Autodesk Inventor part; units mm, degrees
ref_plane "Work Plane1" through (0, 80, 0) normal (-0.7071, 0, 0.7071) x (0, -1, 0)
ref_plane "YZ Plane" through (0, 0, 0) normal (1, 0, 0) x (0, 1, 0)
ref_plane "XZ Plane" through (0, 0, 0) normal (0, 1, 0) x (-1, 0, 0)
sketch "Sketch1" plane through (0, 0, 0) normal (0, 0, 1) x (1, 0, 0)
  line L0 (0, 0) -> (200, 0)
  line L1 (200, 0) -> (200, 80)
  line L2 (200, 80) -> (0, 80)
  line L3 (0, 80) -> (0, 0)
  dimension "d0" = 200
  dimension "d1" = 80
extrude "Extrusion1" add sketch "Sketch1" along normal blind 200
sketch "Sketch2" plane through (0, 80, 0) normal (0, 1, 0) x (1, 0, 0)
  line L0 (0, 0) -> (200, 0)
  line L1 (0, 0) -> (0, -200)
  line L2 (10, -20.6066) -> (10, -190)
  line L3 (20.6066, -10) -> (190, -10)
  line L4 (10, -20.6066) -> (10, -25)
  line L5 (20.6066, -10) -> (25, -10)
  line L6 (105.3033, -94.6967) -> (20.6066, -10)
  line L7 (94.6967, -105.3033) -> (10, -20.6066)
  line L8 (190, -10) -> (105.3033, -94.6967)
  line L9 (94.6967, -105.3033) -> (10, -190)
  line L10 (105.3033, -73.4835) -> (153.7868, -25)
  line L11 (94.6967, -105.3033) -> (84.0901, -115.9099)
  line L12 (73.4835, -105.3033) -> (25, -56.8198)
  line L13 (105.3033, -73.4835) -> (56.8198, -25)
  line L14 (153.7868, -25) -> (56.8198, -25)
  line L15 (25, -56.8198) -> (25, -153.7868)
  line L16 (134.3503, -134.3503) -> (91.9239, -176.7767)
  line L17 (63.6396, -148.4924) -> (148.4924, -63.6396)
  line L18 (176.7767, -91.9239) -> (134.3503, -134.3503)
  arc A0 (176.7767, -91.9239) -> (148.4924, -63.6396) centre (162.6346, -77.7817) ccw
  arc A1 (169.7056, -84.8528) -> (155.5635, -70.7107) centre (162.6346, -77.7817) ccw
  line L19 (169.7056, -84.8528) -> (97.1003, -157.4582)
  line L20 (155.5635, -70.7107) -> (82.9581, -143.316)
  line L21 (73.4835, -105.3033) -> (25, -153.7868)
  line L22 (10, -110.6066) -> (25, -110.6066)
  circle A2 centre (17.5, -110.6066) radius 5.5
  circle A3 centre (17.5, -135.6066) radius 5.5
  circle A4 centre (17.5, -85.6066) radius 5.5
  circle A5 centre (17.5, -65.6066) radius 3.5
  circle A6 centre (17.5, -155.6066) radius 3.5
  arc A7 (63.6396, -148.4924) -> (91.9239, -176.7767) centre (77.7817, -162.6346) ccw
  arc A8 (97.1003, -157.4582) -> (82.9581, -143.316) centre (77.7817, -162.6346) ccw
  dimension "d20" = 40
  dimension "d22" = 11
  dimension "d24" = 11
  dimension "d26" = 11
  dimension "d29" = 7
  dimension "d30" = 7
extrude "Extrusion2" add sketch "Sketch2" along normal blind 10
ref_plane "Work Plane1" through (0, 80, 0) normal (-0.7071, 0, 0.7071) x (0, -1, 0)
sketch "Sketch3" plane through (0, 80, 0) normal (-0.7071, 0, 0.7071) x (0, -1, 0)
  line L0 (80, 282.8427) -> (0, 282.8427)
  line L1 (0, 282.8427) -> (0, 207.8427)
  line L2 (0, 141.4214) -> (0, 282.8427)
  line L3 (0, 282.8427) -> (60, 282.8427)
  line L4 (60, 282.8427) -> (0, 207.8427)
  point P0 (80, 0)
  dimension "d33" = 75
  dimension "d34" = 60
extrude "Extrusion3" cut sketch "Sketch3" along normal mid plane 200
fillet "Fillet1" radius 5 3 edges at (25, 85, 56.8198) (73.4835, 85, 105.3033) (25, 85, 153.7868)
sketch "Sketch5" plane through (0, 90, 0) normal (0, 1, 0) x (1, 0, 0)
  point P0 (0, 0)
sketch "Sketch6" plane through (0, 90, 0) normal (0, 1, 0) x (1, 0, 0)
  arc A0 (63.6396, -148.4924) -> (91.9239, -176.7767) centre (77.7817, -162.6346) ccw
  arc A1 (63.6396, -148.4924) -> (91.9239, -176.7767) centre (77.7817, -162.6346) ccw
  arc A2 (169.7056, -84.8528) -> (155.5635, -70.7107) centre (162.6346, -77.7817) ccw
  arc A3 (176.7767, -91.9239) -> (148.4924, -63.6396) centre (162.6346, -77.7817) ccw
  line L0 (148.4924, -63.6396) -> (63.6396, -148.4924)
  line L1 (63.6396, -148.4924) -> (148.4924, -63.6396)
  line L2 (91.9239, -176.7767) -> (176.7767, -91.9239)
  line L3 (91.9239, -176.7767) -> (176.7767, -91.9239)
  point P0 (0, 0)
extrude "Extrusion5" cut sketch "Sketch6" against normal blind 10
sketch "Sketch7" plane through (0, 90, 0) normal (0, 1, 0) x (1, 0, 0)
  line L0 (105.3033, -94.6967) -> (20.6066, -10)
  line L1 (20.6066, -10) -> (105.3033, -94.6967)
  line L2 (190, -10) -> (105.3033, -94.6967)
  line L3 (105.3033, -94.6967) -> (190, -10)
  line L4 (190, -10) -> (20.6066, -10)
  point P0 (0, 0)
extrude "Extrusion6" cut sketch "Sketch7" against normal blind 10
sketch "Sketch8" plane through (0, 80, 0) normal (0, 1, 0) x (1, 0, 0)
  line L0 (200, 0) -> (0, 0)
  line L1 (0, 0) -> (20.645, 0)
  line L2 (20.645, 0) -> (20.645, -20)
  line L3 (20.645, -20) -> (126.7111, -126.066)
  line L4 (20.645, -20) -> (170.645, -20) construction
  line L5 (126.7111, -126.066) -> (200, -52.7771)
  line L6 (200, 0) -> (200, -93.934)
  line L7 (20.645, 0) -> (200, 0)
  line L8 (200, -52.7771) -> (200, 0)
  dimension "d45" = 20
  dimension "d46" = 150
  dimension "d47" = 45
extrude "Extrusion7" cut sketch "Sketch8" against normal blind 10
fillet "Fillet2" radius 20 2 edges at (126.7111, 75, 126.066) (20.645, 75, 20)
sketch "Sketch9" plane through (0, 70, 0) normal (0, 1, 0) x (1, 0, 0)
  arc A0 (112.5689, -111.9239) -> (140.8532, -111.9239) centre (126.7111, -97.7817) ccw
  arc A1 (117.4902, -106.2213) -> (135.9319, -106.2213) centre (126.7111, -97.7817) ccw
  arc A2 (20.645, -11.7157) -> (26.5029, -25.8579) centre (40.645, -11.7157) ccw
  arc A3 (28.145, -11.7157) -> (31.8071, -20.5555) centre (40.645, -11.7157) ccw
  line L0 (117.4902, -106.2213) -> (31.8071, -20.5555)
  line L1 (135.9319, -106.2213) -> (226.547, -106.2213) construction
  line L2 (200, 0) -> (200, -52.7771)
  line L3 (200, 0) -> (192.5, 0)
  line L4 (20.645, 0) -> (200, 0)
  line L5 (192.5, -7.5) -> (192.5, -49.6532)
  line L6 (200, 0) -> (200, -7.5)
  line L7 (192.5, -7.5) -> (28.145, -7.5)
  line L8 (28.145, -11.7157) -> (28.145, -7.5)
  line L9 (135.9319, -106.2213) -> (192.5, -49.6532)
  line L10 (200, -42.1532) -> (200.0065, -42.1467)
  line L11 (126.7111, -97.7817) -> (126.7111, -85.2817)
  circle A4 centre (126.7111, -97.7817) radius 12.5
  point P0 (0, 0)
  dimension "d51" = 25
  dimension "d52" = 25
  dimension "d54" = 7.5
  dimension "d55" = 7.5
extrude "Extrusion8" cut sketch "Sketch9" against normal blind 10 contours L0 A3 L8 L7 L5 L9 A4
sketch "Sketch10" plane through (0, 70, 0) normal (0, 1, 0) x (1, 0, 0)
  arc A0 (135.9319, -106.2213) -> (117.4902, -106.2213) centre (126.7111, -97.7817) ccw
  circle A1 centre (126.7111, -97.7817) radius 20
  point P0 (0, 0)
extrude "Extrusion9" add sketch "Sketch10" along normal blind 10 and the other way blind 10
sketch "Sketch11" plane through (0, 80, 200) normal (0, 1, 0) x (1, 0, 0)
  arc A0 (146.5879, 104.4347) -> (106.834, 104.4327) centre (126.7111, 102.2183) ccw
  line L0 (126.7111, 102.2183) -> (112.5689, 116.3604)
  line L1 (126.7111, 102.2183) -> (146.7111, 102.2183) construction
  line L2 (112.5689, 116.3604) -> (98.4268, 102.2183)
  line L3 (112.5689, 88.0761) -> (26.5029, 174.1421)
  line L4 (140.8532, 116.3604) -> (154.9953, 102.2183)
  line L5 (200, 147.2229) -> (140.8532, 88.0761)
  arc A1 (112.5689, 88.0761) -> (140.8532, 88.0761) centre (126.7111, 102.2183) ccw
  arc A2 (140.8532, 116.3604) -> (112.5689, 116.3604) centre (126.7111, 102.2183) ccw
  line L6 (112.5689, 88.0761) -> (98.4268, 102.2183)
  line L7 (154.9953, 102.2183) -> (140.8532, 88.0761)
  point P0 (0, 200)
  dimension "d62" = 135
extrude "Extrusion10" add sketch "Sketch11" against normal blind 20
fillet "Fillet3" radius 10 2 edges at (103.7373, 65, 92.4712) (149.6834, 65, 92.4698)
sketch "Sketch12" plane through (0, 70, 0) normal (0, 1, 0) x (1, 0, 0)
  arc A0 (140.8532, -83.6396) -> (112.5689, -83.6396) centre (126.7111, -97.7817) ccw
  line L0 (107.8365, -77.7817) -> (93.1316, -92.4866)
  line L1 (98.4268, -97.7817) -> (26.5029, -25.8579)
  line L2 (146.1565, -78.3363) -> (160.2986, -92.4784)
  line L3 (200, -52.7771) -> (154.9953, -97.7817)
  line L4 (160.2986, -92.4784) -> (127.5069, -125.2702)
  line L5 (127.5069, -125.2702) -> (93.9274, -91.6908)
  arc A1 (146.1565, -78.3363) -> (106.7111, -78.9072) centre (126.7111, -97.7817) ccw
  point P0 (0, 0)
extrude "Extrusion11" add sketch "Sketch12" against normal blind 20 contours A1 L2 L3 L4 L5 L0
fillet "Fillet4" radius 5 2 edges at (98.6681, 65, 86.9501) (154.7622, 65, 86.942)
fillet "Fillet5" radius 5 2 edges at (98.4268, 75, 97.7817) (154.9953, 75, 97.7817)
fillet "Fillet6" radius 5 3 edges at (192.5, 65, 7.5) (192.5, 65, 49.6532) (28.145, 65, 7.5)
sketch "Sketch13" plane through (0, 60, 0) normal (0, 1, 0) x (1, 0, 0)
  line L0 (200, 0) -> (200, -52.7771)
  line L1 (200, 0) -> (200, -35)
  line L2 (200, -35) -> (160, -35)
  circle A0 centre (160, -35) radius 20
  circle A1 centre (160, -35) radius 10
  point P0 (0, 0)
  dimension "d72" = 35
  dimension "d73" = 40
  dimension "d74" = 40
  dimension "d75" = 20
extrude "Extrusion12" add sketch "Sketch13" along normal blind 20
fillet "Fillet7" radius 10 3 edges at (94.6967, 85, 105.3033) (10, 85, 20.6066) (10, 85, 190)
fillet "Fillet8" radius 3 6 edges at (28.0866, 80, 146.3351) (51.7417, 80, 127.045) (71.4124, 80, 105.3033) (51.7417, 80, 83.5616) (28.0866, 80, 64.2715) (25, 80, 105.3033)
sketch "Sketch14" plane through (160, 80, 35) normal (0, 1, 0) x (1, 0, 0)
  circle A0 centre (0, 0) radius 20
  circle A1 centre (-20, 0) radius 5.5
  point P0 (-160, 35)
  dimension "d80" = 11
extrude "Extrusion13" cut sketch "Sketch14" against normal blind 20 contours A1 A0 | A0 A1 picked at (-18.1103, 0) picked at (-21.777, 0)
sketch "Sketch15" plane through (0, 80, 200) normal (0, 1, 0) x (1, 0, 0)
  line L0 (87.6256, 87.6256) -> (27.0711, 27.0711)
  line L1 (27.0711, 27.0711) -> (87.6256, 87.6256)
  line L2 (87.6256, 87.6256) -> (27.0711, 27.0711)
  line L3 (36.3259, 18.3055) -> (116.2946, 98.2741)
  line L4 (116.2946, 98.2741) -> (18.0204, 0)
  line L5 (116.2946, 98.2741) -> (141.0433, 73.5254)
  line L6 (141.0433, 73.5254) -> (67.5179, 0)
  line L7 (93.934, 0) -> (0, 0)
  line L8 (67.5179, 0) -> (18.0204, 0)
  point P0 (0, 200)
  dimension "d83" = 35
extrude "Extrusion14" cut sketch "Sketch15" against normal blind 10
fillet "Fillet9" radius 10 2 edges at (116.2946, 75, 101.7259) (141.0433, 75, 126.4746)
sketch "Sketch17" plane through (0, 90, 0) normal (0, 1, 0) x (1, 0, 0)
  circle A0 centre (17.5, -110.6066) radius 5.5
  circle A1 centre (17.5, -110.6066) radius 5.5
  circle A2 centre (17.5, -135.6066) radius 5.5
  circle A3 centre (17.5, -135.6066) radius 5.5
  circle A4 centre (17.5, -85.6066) radius 5.5
  circle A5 centre (17.5, -85.6066) radius 5.5
  circle A6 centre (17.5, -65.6066) radius 3.5
  circle A7 centre (17.5, -65.6066) radius 3.5
  circle A8 centre (17.5, -155.6066) radius 3.5
  circle A9 centre (17.5, -155.6066) radius 3.5
  point P0 (0, 0)
hole "Hole1" at (17.5, 90, 85.6066) at (17.5, 90, 110.6066) at (17.5, 90, 135.6066) direction (0, -1, 0) diameter 11 depth 25 tip angle 118
sketch "Sketch18" plane through (0, 90, 0) normal (0, 1, 0) x (1, 0, 0)
  circle A0 centre (17.5, -65.6066) radius 3.5
  circle A1 centre (17.5, -65.6066) radius 3.5
  circle A2 centre (17.5, -155.6066) radius 3.5
  circle A3 centre (17.5, -155.6066) radius 3.5
  point P0 (0, 0)
hole "Hole2" at (17.5, 90, 65.6066) at (17.5, 90, 155.6066) direction (0, -1, 0) diameter 11 depth 25 tip angle 118
thread "Thread1"
thread "Thread2"
thread "Thread3"
properties part number "proyecto"
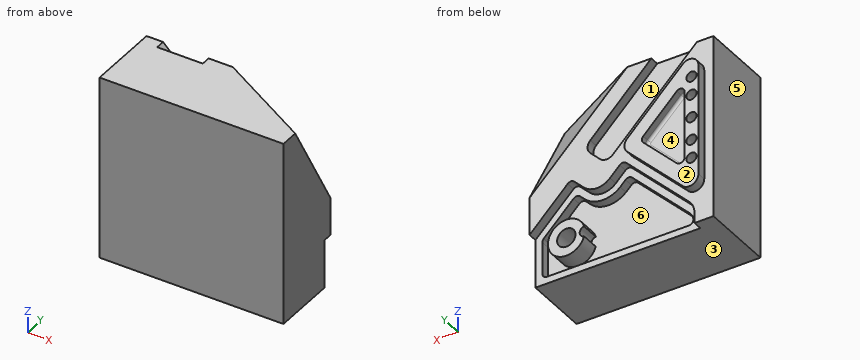
Verification items for the finished model (mm, model axes). Face numbers are marked on the shaded views. A direction names the side the tool comes from. Give positions to 0.01 mm unless a question says otherwise; leave off trailing zeros. Order: outer loops, then holes, each group sorted by start corner. A loop starts at its lowest first (then second) coordinate and runs counter-clockwise, first axis right, second up. Notation, with made-up numbers: M 83,-16.5 L 108,-16.5 A6 cw 108,-10.5 Z; hole C -25.75,-2 d2. An arc over 180 degrees is marked long. Answer in a Markdown table with one row per item. Add a question column.
Item 1: Gauge pin test, flat ends, axial feed: pin 1 (4 mm diameter, centred on y = 74.5, z = 165, fed in from -X); pin 2 (2 mm diameter, centred on x = 151, y = 79, fed in from -Z); pin 3 (16 mm diameter, centred on x = 160, z = 36, fed in from +Y); pin 4 (20 mm diameter, centred on x = 44.5, z = 115.5, fed in from +Y). Record the tip position at first contact, or that the pin passes through.
Item 2: Tool access check on the marked faces 1 and 2. Record the directions out of +Z, -Z, +X, -X, +Y, -Y that give a thin tool (end or side, any length) a straight path to the whole face; none if there is none.
Item 3: Scan lines: probe 1 along Z at (x, y) = (17.5, 70.5); probe 2 along Y at (x, z) = (192.5, 89.5); probe 3 along Y at (x, z) = (178, 25.5). Record each from-to range of solid material in increasing order. Write a range as from..to.
Item 4: Section check C-C, the plane y = 48. Enter the section's corners in (x, z), and give its area (3 significant figures).
Item 5: Section check A-A, the plane y = 76. State how many separate pieces and enclosed holes the cut face has, and give its area (3 significant figures).
Item 6: Mould release check, pull along X, two halves, no side actions. Record for the marked faces 3, 4, 5 and 6: released by +X, released by -X, zero draft, split by the parting line, or undercut.
Item 7: Section check B-B, the plane z = 185.5. Enter the section's corners in (x, y), and give its area (3 significant figures).
Filled sheet:
| question | item | result |
|---|---|---|
| 1 | pin 1 | stops at x = 0 |
| 1 | pin 2 | stops at z = 16.67 |
| 1 | pin 3 | stops at y = 60 |
| 1 | pin 4 | stops at y = 80 |
| 2 | face 1 | +Y |
| 2 | face 2 | +Z, -Z, +X, -X, +Y |
| 3 | probe 1 | z = 0..60.11, 71.11..80.11, 91.11..105.11, 116.11..130.11, 141.11..150.11, 161.11..200 |
| 3 | probe 2 | y = 0..80 |
| 3 | probe 3 | y = 0..60 |
| 4 | outline | M 0,0 L 200,0 L 200,150.5 L 150.5,200 L 0,200 Z |
| 4 | area | 38,800 mm^2 |
| 5 | separate pieces | 2 |
| 5 | enclosed holes | 6 |
| 5 | area | 18,500 mm^2 |
| 6 | face 3 | zero draft |
| 6 | face 4 | undercut |
| 6 | face 5 | released by -X |
| 6 | face 6 | undercut |
| 7 | outline | M 0,0 L 200,0 L 200,28.2 L 108.43,80 L 82.02,80 L 82.02,70 L 32.52,70 L 32.52,80 L 0,80 Z |
| 7 | area | 13,100 mm^2 |
